Geometry check sheet. Reference: drawing and pictorial views, mm from the part's lowest x, y, z. A direction names the side the tool comes from. Round coordinates to 2 decimals unless told otherwise and drop trailing zeros. Order: outer loops, then holes, each group sorted by start corner. A loop starts at its lowest first (then second) coordinate and runs counter-clockwise, first axis right, second up.
(1) Sectioned sample at B-B (z = 1.25). Record the boundary of the cut face in (x, y) (1 decimal), plus the area to 3 significant figures.
(2) Set-up check for the marked faces 1 and 2: record each of +Z, -Z, +X, -X, +Y, -Y from which the full face is reachable in a straight line by a thin tool's end or side.
(3) Sectioned sample at C-C (z = 4). Record the boundary of the cut face in (x, y) (1 decimal), plus the area to 3 significant figures.
(4) Material ranges on line 1 along X through (y, z) = (20, 1.5) (1 decimal); line 2 along Z through (x, y) = (16.5, 5) (1 decimal); line 3 along Y through (x, z) = (12.5, 5) (1 decimal), recorded low to high.
(5) Sectioned sample at D-D (z = 10.75). Record the boundary of the cut face in (x, y).
(6) Go/stop test with flat-tipped pins: pin 1 (1 mm diameter, centred on x = 35, z = 5.5, fed in from -Y); pin 2 (6 mm diameter, centred on x = 32.5, z = 3.5, fed in from +Y); pin 3 (1 mm diameter, centred on x = 21, y = 19.5, fed in from -Z); pin 4 (4 mm diameter, centred on x = 19.99, y = 3.16, fed in from +Z) (3 decimals). Record where each tip stops, or that it passes through.
(7) Sectioned sample at A-A (x = 36.5). Record the boundary of the cut face in (y, z) (1 decimal).
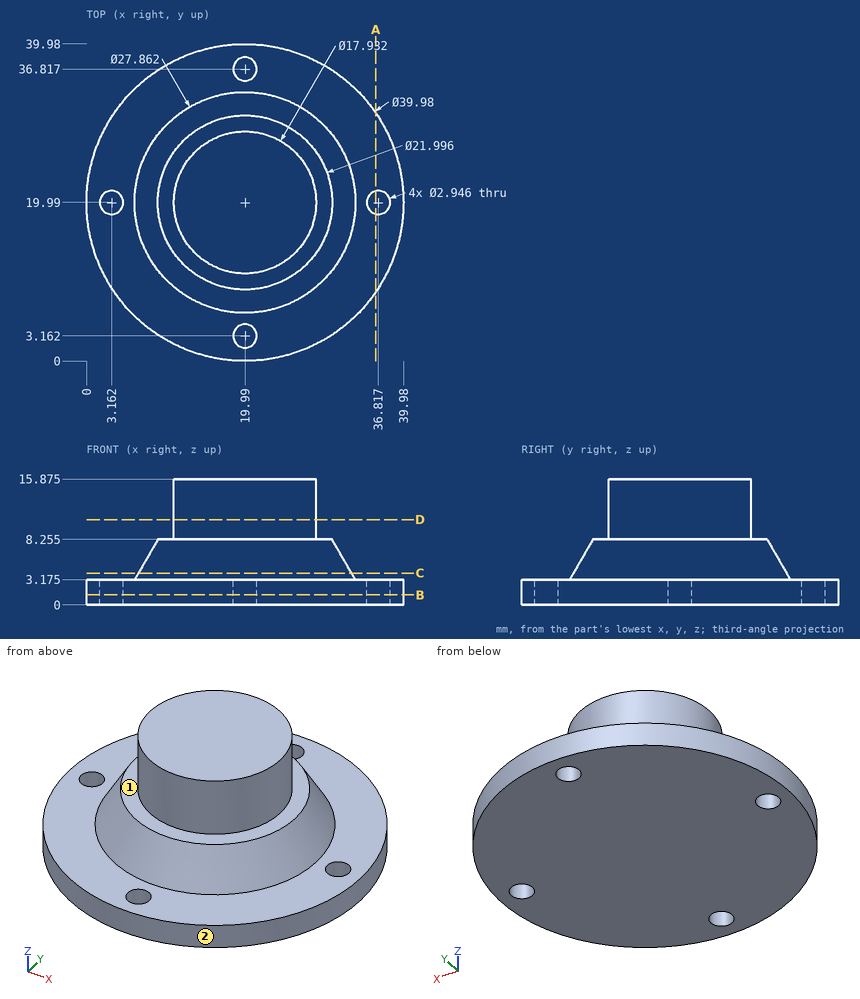
Answer below:
1. outline: circle Ø40 at (20, 20); hole circle Ø2.9 at (3.2, 20); hole circle Ø2.9 at (20, 3.2); hole circle Ø2.9 at (20, 36.8); hole circle Ø2.9 at (36.8, 20)
1. area: 1,230 mm2
2. face 1: +Z
2. face 2: +Z, -Z
3. outline: circle Ø26.9 at (20, 20)
3. area: 569 mm2
4. line 1: x = 0 to 1.7, 4.6 to 35.3, 38.3 to 40
4. line 2: z = 0 to 3.2
4. line 3: y = 9.5 to 30.5
5. outline: circle Ø17.93 at (19.99, 19.99)
6. pin 1: passes through
6. pin 2: stops at y = 37.56
6. pin 3: stops at z = 0
6. pin 4: stops at z = 3.175
7. outline: (8.7, 0) - (18.6, 0) - (18.6, 3.2) - (8.7, 3.2) - close; (21.4, 0) - (31.3, 0) - (31.3, 3.2) - (21.4, 3.2) - close
